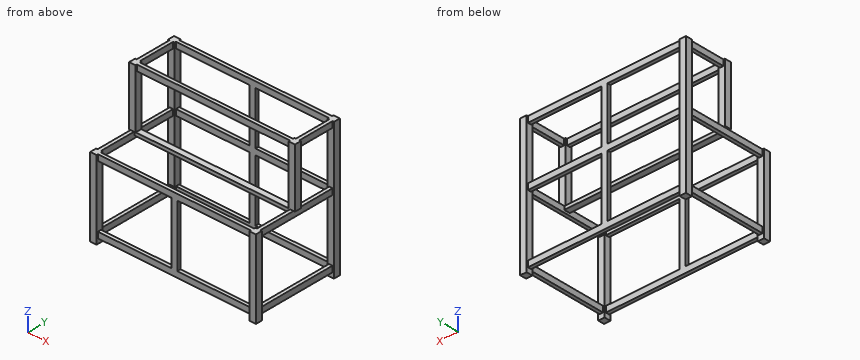
from build123d import *

# Parameters (mm, degrees)
F0_W      = 1700
F0_H      = 800
F1_DEPTH  = 65
F2_W      = 1570
F2_H      = 15
F3_DEPTH  = 800.001
F4_W      = 1570
F4_H      = 50
F4_W_2    = 755
F4_H_2    = 630
F5_DEPTH  = 50.001
F6_W      = 35
F6_H      = 60
F7_DEPTH  = 800
F8_W      = 65
F8_H      = 65
F9_DEPTH  = 1400
F10_W     = 35
F10_H     = 60
F11_DEPTH = 1570
F12_W     = 60
F12_H     = 35
F13_DEPTH = 1230
F14_W     = 60
F14_H     = 35
F15_DEPTH = 1600
F16_W     = 65
F16_H     = 65
F17_DEPTH = 600
F18_W     = 35
F18_H     = 60
F19_DEPTH = 367.5
F20_W     = 35
F20_H     = 60
F21_DEPTH = 1570


with BuildPart() as f1:
    # F0 (on Front) → F1 (new body)
    with BuildSketch(Plane.XZ):
        with Locations((850, 400)):
            Rectangle(F0_W, F0_H)
    extrude(amount=F1_DEPTH)

    # F2 (on face) → F3 (cut, through all)
    with BuildSketch(Plane.XY.offset(800)):
        with Locations((850, -57.5)):
            Rectangle(F2_W, F2_H)
        with Locations((850, -7.5)):
            Rectangle(F2_W, F2_H)
    extrude(amount=-F3_DEPTH, mode=Mode.SUBTRACT)

    # F4 (on face) → F5 (cut, through all)
    with BuildSketch(Plane.XZ.offset(50)):
        with Locations((850, 25)):
            Rectangle(F4_W, F4_H)
        with Locations((1257.5, 425)):
            Rectangle(F4_W_2, F4_H_2)
        with Locations((442.5, 425)):
            Rectangle(F4_W_2, F4_H_2)
    extrude(amount=-F5_DEPTH, mode=Mode.SUBTRACT)

    # F6 (on face) → F7 (join)
    with BuildSketch(Plane(origin=(0, 0, 0), x_dir=(-1, 0, 0), z_dir=(0, 1, 0))):
        with Locations((-1667.5, 770)):
            Rectangle(F6_W, F6_H)
        with Locations((-1667.5, 80)):
            Rectangle(F6_W, F6_H)
        with Locations((-32.5, 770)):
            Rectangle(F6_W, F6_H)
        with Locations((-32.5, 80)):
            Rectangle(F6_W, F6_H)
    extrude(amount=F7_DEPTH)

    # F8 (on face) → F9 (join)
    with BuildSketch(Plane(origin=(0, 0, 0), x_dir=(1, 0, 0), z_dir=(0, 0, -1))):
        with Locations((1667.5, -832.5)):
            Rectangle(F8_W, F8_H)
        with Locations((32.5, -832.5)):
            Rectangle(F8_W, F8_H)
    extrude(amount=-F9_DEPTH)

    # F10 (on face) → F11 (join)
    with BuildSketch(Plane.YZ.offset(65)):
        with Locations((832.5, 1370)):
            Rectangle(F10_W, F10_H)
        with Locations((832.5, 80)):
            Rectangle(F10_W, F10_H)
        with Locations((832.5, 770)):
            Rectangle(F10_W, F10_H)
    extrude(amount=F11_DEPTH)

    # F12 (on face) → F13 (join, through all)
    with BuildSketch(Plane.XY.offset(110)):
        with Locations((850, 832.5)):
            Rectangle(F12_W, F12_H)
    extrude(amount=F13_DEPTH)

    # F14 (on face) → F15 (join, through all)
    with BuildSketch(Plane.YZ.offset(50)):
        with Locations((400, 782.5)):
            Rectangle(F14_W, F14_H)
    extrude(amount=F15_DEPTH)

    # F16 (on face) → F17 (join)
    with BuildSketch(Plane.XY.offset(800)):
        with Locations((32.5, 400)):
            Rectangle(F16_W, F16_H)
        with Locations((1667.5, 400)):
            Rectangle(F16_W, F16_H)
    extrude(amount=F17_DEPTH)

    # F18 (on face) → F19 (join, through all)
    with BuildSketch(Plane.XZ.offset(-800)):
        with Locations((1667.5, 1370)):
            Rectangle(F18_W, F18_H)
        with Locations((32.5, 1370)):
            Rectangle(F18_W, F18_H)
    extrude(amount=F19_DEPTH)

    # F20 (on face) → F21 (join, through all)
    with BuildSketch(Plane.YZ.offset(65)):
        with Locations((400, 1370)):
            Rectangle(F20_W, F20_H)
    extrude(amount=F21_DEPTH)


solid = f1.part
CAD build for the part. Positions are in the model's coordinates, mm. Give positions to 0.01 mm unless a question says otherwise; leave off trailing zeros. Write each loop counter-clockwise with the first axis right and the second up, starting at its lowest first coordinate (ties: lowest second). Pieces come first, ordered by that corner, then holes. Notation, with made-up numbers: (-38.75, 46) - (-32.75, 46) arc R29 cw to (-32.75, 69) - close; hole circle Ø6 at (18.5, -6.5). An arc over 180 degrees is marked (long way). Put each result on its own line as item: value.
(1) Wall check: L1, parallel to Y at x = 1225, z = 101; L2, parallel to X at y = 32, z = 78; L3, parallel to Z at x = 1474, y = 388. Give the ranges that are in metal, low to high.
Working result:
L1: -50 to -15, 815 to 850
L2: 15 to 50, 1650 to 1685
L3: 765 to 800, 1340 to 1400
(2) Saw through at A-A (z = 872). List the corners of the cut face in (x, y), then the cut area to 3 significant figures.
Working result:
outline: (0, 367.5) - (65, 367.5) - (65, 432.5) - (0, 432.5) - close; (0, 800) - (65, 800) - (65, 865) - (0, 865) - close; (820, 815) - (880, 815) - (880, 850) - (820, 850) - close; (1635, 367.5) - (1700, 367.5) - (1700, 432.5) - (1635, 432.5) - close; (1635, 800) - (1700, 800) - (1700, 865) - (1635, 865) - close
area: 19,000 mm^2
(3) Saw through at B-B (y = 759). List the corners of the cut face in (x, z).
Working result:
outline: (15, 50) - (50, 50) - (50, 110) - (15, 110) - close; (15, 740) - (50, 740) - (50, 800) - (15, 800) - close; (15, 1340) - (50, 1340) - (50, 1400) - (15, 1400) - close; (1650, 50) - (1685, 50) - (1685, 110) - (1650, 110) - close; (1650, 740) - (1685, 740) - (1685, 800) - (1650, 800) - close; (1650, 1340) - (1685, 1340) - (1685, 1400) - (1650, 1400) - close
(4) Drop flat-ended pins along their axis: pin 1 Ø16.5 at (x, y) = (1693.5, 396) entering from -Z; pin 2 Ø17.5 at (x, y) = (363.5, 827.5) entering from -Z; pin 3 Ø2 at (x, y) = (1453.5, 371) entering from +Z. Give the stop position or say it passes through.
Working result:
pin 1: z = 800
pin 2: z = 50
pin 3: z = 800
(5) Saw through at C-C (x = 477). List the corners of the cut face in (y, z), then the cut area to 3 significant figures.
Working result:
outline: (-50, 50) - (-15, 50) - (-15, 110) - (-50, 110) - close; (-50, 740) - (-15, 740) - (-15, 800) - (-50, 800) - close; (370, 765) - (430, 765) - (430, 800) - (370, 800) - close; (382.5, 1340) - (417.5, 1340) - (417.5, 1400) - (382.5, 1400) - close; (815, 50) - (850, 50) - (850, 110) - (815, 110) - close; (815, 740) - (850, 740) - (850, 800) - (815, 800) - close; (815, 1340) - (850, 1340) - (850, 1400) - (815, 1400) - close
area: 14,700 mm^2
(6) Saw through at D-D (y = 119). List the corners of the cut face in (x, z), then the cut area to 3 significant figures.
Working result:
outline: (15, 50) - (50, 50) - (50, 110) - (15, 110) - close; (15, 740) - (50, 740) - (50, 800) - (15, 800) - close; (1650, 50) - (1685, 50) - (1685, 110) - (1650, 110) - close; (1650, 740) - (1685, 740) - (1685, 800) - (1650, 800) - close
area: 8,400 mm^2
